```python
from build123d import *

# Parameters (mm, degrees)
PAD_DEPTH     = 15
SKETCH001_R   = 30
POCKET_DEPTH  = 5
SKETCH002_R   = 3.4
HOLE_DEPTH    = 15.001
FILLET_R      = 5
SKETCH003_R   = 2.5
HOLE001_DEPTH = 15.001


with BuildPart() as part:
    # Sketch → Pad (new body)
    with BuildSketch(Plane.XY):
        with BuildLine():
            Line((50, 0), (500, 0))
            ThreePointArc((500, 0), (535.355339, 14.644661), (550, 50))
            Line((550, 50), (550, 140))
            Line((470, 140), (550, 140))
            Line((470, 320), (470, 140))
            Line((550, 320), (470, 320))
            Line((550, 320), (550, 550))
            ThreePointArc((550, 550), (535.355339, 585.355339), (500, 600))
            Line((500, 600), (50, 600))
            ThreePointArc((50, 600), (14.644661, 585.355339), (0, 550))
            Line((0, 550), (0, 320))
            Line((0, 320), (80, 320))
            Line((80, 320), (80, 140))
            Line((80, 140), (0, 140))
            Line((0, 140), (0, 50.00011))
            ThreePointArc((0, 50.00011), (14.644622, 14.6447), (50, 0))
        make_face()
    extrude(amount=PAD_DEPTH)

    # Sketch001 (on Face17 of Pad) → Pocket (cut)
    with BuildSketch(Plane(origin=(0, 0, 0), x_dir=(1, 0, 0), z_dir=(0, 0, -1))):
        with Locations((500, -60)):
            Circle(SKETCH001_R)
        with Locations((50, -60)):
            Circle(SKETCH001_R)
        with Locations((500, -530)):
            Circle(SKETCH001_R)
        with Locations((50, -530)):
            Circle(SKETCH001_R)
    extrude(amount=-POCKET_DEPTH, mode=Mode.SUBTRACT)

    # Sketch002 (on Face4 of Pocket) → Hole (cut, through all)
    with BuildSketch(Plane(origin=(0, 0, 0), x_dir=(1, 0, 0), z_dir=(0, 0, -1))):
        with Locations((50, -60)):
            Circle(SKETCH002_R)
        with Locations((500, -60)):
            Circle(SKETCH002_R)
        with Locations((500, -530)):
            Circle(SKETCH002_R)
        with Locations((50, -530)):
            Circle(SKETCH002_R)
    extrude(amount=-HOLE_DEPTH, mode=Mode.SUBTRACT)

    # Fillet
    fillet_edges = [part.edges().sort_by_distance(p)[0] for p in [
        (550, 320, 7.5),
        (550, 140, 7.5),
        (470, 320, 7.5),
        (470, 140, 7.5),
        (80, 140, 7.5),
        (0, 140, 7.5),
        (0, 320, 7.5),
        (80, 320, 7.5),
    ]]
    fillet(fillet_edges, radius=FILLET_R)

    # Sketch003 (on Face5 of Fillet) → Hole001 (cut, through all)
    with BuildSketch(Plane.XY.offset(15)):
        with Locations((30, 425)):
            Circle(SKETCH003_R)
        with Locations((520, 425)):
            Circle(SKETCH003_R)
        with Locations((65, 110)):
            Circle(SKETCH003_R)
        with Locations((485, 110)):
            Circle(SKETCH003_R)
    extrude(amount=-HOLE001_DEPTH, mode=Mode.SUBTRACT)


solid = part.part
```
Verification items for the finished model (mm, model axes). A direction names the side the tool comes from. Coordinates: 2 decimals unless noted, no trailing zeros. Order: outer loops, then holes, each group sorted by start corner. A loop starts at its lowest first (then second) coordinate and runs counter-clockwise, first axis right, second up. Notation, with made-up numbers: (56.5, 22.5) -> (80.5, 22.5) arc R22 ccw to (80.5, 41.5) -> close; hole circle Ø11 at (-37.75, 13.5). An arc over 180 degrees is marked (long way). Put each result on its own line as item: value. Start each with the question number.
1) Material ranges on L1, parallel to Y at x = 50, z = 2.3; L2, parallel to Y at x = 500, z = 7.5; L3, parallel to X at y = 530, z = 8.5, recorded low to high.
2) Tool access check on faces 1 (the flat face through (510, 320, 7)), 2 (the flat face through (56, 60, 5)), 3 (the flat face through (40, 320, 7)). Record the directions out of +Z, -Z, +X, -X, +Y, -Y that give a thin tool (end or side, any length) a straight path to the whole face; none if there is none.
3) Cross-section at B-B (y = 174). Enter the section's corners in (x, z).
4) Go/stop test with flat-tipped pins: pin 1 (4.5 mm diameter, centred on y = 269.5, z = 4, fed in from -X); pin 2 (4 mm diameter, centred on x = 520, y = 425, fed in from -Z); pin 3 (8 mm diameter, centred on x = 500, y = 60, fed in from -Z). Record where each tip stops, or that it passes through.
5) Cross-section at A-A (z = 8.75). State how many separate pieces and enclosed holes the cut face has, plus the area to 3 significant figures.
6) Release check for a two-part mould opening along X. For faces 4 (the cylindrical face through (46.095, 500.255, 2.465)), 5 (the flat face through (80, 231, 7)), 6 (the flat face through (506, 530, 5)), 7 (the flat face through (510, 140, 7)) record: pulls with the +X half, pulls with the -X half, needs draft (parallel to the pull), parting line crosses it, or undercut.
Geometry check:
1. L1: y = 0 to 30, 90 to 140, 320 to 500, 560 to 600
1. L2: y = 0 to 56.6, 63.4 to 140, 320 to 526.6, 533.4 to 600
1. L3: x = 0 to 46.6, 53.4 to 496.6, 503.4 to 550
2. face 1: +Z, -Z, +X
2. face 2: -Z
2. face 3: +Z, -Z, -X
3. outline: (80, 0) -> (470, 0) -> (470, 15) -> (80, 15) -> close
4. pin 1: stops at x = 80
4. pin 2: passes through
4. pin 3: stops at z = 5
5. separate pieces: 1
5. enclosed holes: 8
5. area: 299,000 mm^2
6. face 4: undercut
6. face 5: pulls with the -X half
6. face 6: undercut
6. face 7: needs draft
